Build history of the part. All positions in model axes, mm. A direction names the side the tool comes from. Round coordinates to 2 decimals unless told otherwise and drop trailing zeros. Loops run counter-clockwise (first coordinate to the right, second up) from the corner with the lowest first, then second, coordinate; pieces in that order, holes last. Notation, with made-up numbers: (57, 2.25) - (76, 2.25) arc R15 cw to (76, 20.25) - close; hole circle Ø6 at (-37, 17). An arc over 180 degrees is marked (long way). Put each result on its own line as item: value. Start each with the question number.
Autodesk Fusion 360 part; units mm, degrees
sketch "Esquisse1" plane through (0, 0, 0) normal (0, 1, 0) x (1, 0, 0)
  line L0 (0, 0) -> (150, 0)
  line L1 (150, 0) -> (150, -35)
  line L2 (150, -35) -> (0, -35)
  line L3 (0, -35) -> (0, 0)
  line L4 (75, -35) -> (75, -60) construction
  line L5 (0, 0) -> (150, 0)
  line L6 (150, 0) -> (150, 2.5)
  line L7 (150, 2.5) -> (0, 2.5)
  line L8 (0, 2.5) -> (0, 0)
  line L9 (150, -35) -> (152.5, -35)
  line L10 (152.5, -35) -> (152.5, 2.5)
  line L11 (152.5, 2.5) -> (150, 2.5)
  line L12 (150, 2.5) -> (150, -35)
  line L13 (0, -35) -> (-2.5, -35)
  line L14 (-2.5, -35) -> (-2.5, 2.5)
  line L15 (-2.5, 2.5) -> (0, 2.5)
  line L16 (0, 2.5) -> (0, -35)
  line L17 (-2.5, -35) -> (71.93, -59.0097)
  line L18 (78.07, -59.0097) -> (152.5, -35)
  arc A0 (71.93, -59.0097) -> (78.07, -59.0097) centre (75, -49.4926) ccw
  point P0 (75, -35)
  dimension "d6" = 150
  dimension "d7" = 35
  dimension "d8" = 25
  dimension "d13" = 150
  dimension "d14" = 2.5
  dimension "d15" = 2.5
  dimension "d16" = 37.5
  dimension "d17" = 2.5
  dimension "d18" = 37.5
  dimension "d19" = 10
extrude "Extrusion2" add sketch "Esquisse1" along normal blind 2.5 contours L0 L1 L2 L3 L5 L12 L16 | L2 L9 L13 L17 L18 A0
extrude "Extrusion3" add sketch "Esquisse1" along normal blind 70 contours L0 L5 L6 L7 L8 L12 L16 | L3 L8 L13 L14 L15 L16 | L1 L6 L9 L10 L11 L12
ref_plane "Plan de construction1" through (75, 70, 16.25) normal (0, 1, 0) x (0, 0, 1)
sketch "Esquisse2" plane through (75, 70, 16.25) normal (0, 1, 0) x (1, 0, 0)
  line L0 (-75, 16.25) -> (-75, -18.75)
  line L1 (-75, -18.75) -> (-77.5, -18.75)
  line L2 (-77.5, -18.75) -> (-3.07, -42.7597)
  arc A0 (-3.07, -42.7597) -> (3.07, -42.7597) centre (0, -33.2426) ccw
  line L3 (3.07, -42.7597) -> (77.5, -18.75)
  line L4 (77.5, -18.75) -> (75, -18.75)
  line L5 (75, -18.75) -> (75, 16.25)
  line L6 (75, 16.25) -> (-75, 16.25)
  line L7 (75, -18.75) -> (-75, -18.75)
  line L8 (-75, -18.75) -> (-75, 16.25)
  line L9 (-75, 16.25) -> (75, 16.25)
  line L10 (75, 16.25) -> (75, -18.75)
  line L11 (75, -1.25) -> (-75, -1.25) construction
  line L12 (75, -1.25) -> (25, -1.25) construction
  line L13 (-75, -1.25) -> (-25, -1.25) construction
  circle A1 centre (25, -1.25) radius 2.25
  circle A2 centre (-25, -1.25) radius 2.25
  point P0 (75, -1.25)
  point P1 (-75, -1.25)
  dimension "d27" = 50
  dimension "d28" = 50
  dimension "d30" = 4.5
  dimension "d31" = 4.5
extrude "Extrusion4" add sketch "Esquisse2" against normal blind 2.5 contours L0 L5 L6 L7 L8 L9 L10 | A1 | A2
extrude "Extrusion5" cut sketch "Esquisse2" against normal blind 2.5 contours A1 | A2
equation "bagWidth = 150 mm"
equation "bagThickness = 65 mm"
equation "dispenserBorderHeight = 35 mm"
equation "dispenserTriangleHeight = 25 mm"
equation "dispenserThickness = 2.5 mm"
equation "d6 = bagWidth"
equation "d7 = dispenserBorderHeight"
equation "d8 = dispenserTriangleHeight"
equation "dispenserTriangleRoundCorner = 10 mm"
equation "d13 = bagWidth"
equation "d14 = dispenserThickness"
equation "d15 = dispenserThickness"
equation "d16 = dispenserBorderHeight + dispenserThickness"
equation "d17 = dispenserThickness"
equation "d18 = dispenserBorderHeight + dispenserThickness"
equation "d19 = dispenserTriangleRoundCorner"
equation "d20 = dispenserThickness"
equation "d22 = ( 2 * dispenserThickness ) + bagThickness"
equation "d27 = bagWidth / 3"
equation "d28 = bagWidth / 3"
equation "screwHoleDiameter = 4.5 mm"
equation "d30 = screwHoleDiameter"
equation "d31 = screwHoleDiameter"
1) Slice it at C-C, the plane y = 24. Write the cut outline in (x, z), and give its area (4 significant figures).
2) Slice it at D-D, the plane x = 13. Write the cut outline in (y, z).
3) Slice it at A-A, the plane z = 6. Write the cut outline in (x, y).
4) Drop flat-ended pins along their axis: pin 1 Ø3 at (x, y) = (26, 32.5) entering from +Z; pin 2 Ø3 at (x, z) = (57.5, 45) entering from +Y. Give the stop position or say it passes through.
5) Drill centre lines: line 1 (X direction, y = 68.95, z = 17.5); line 2 (Z direction, x = 100, y = 68.1); line 3 (Y direction, x = 146, z = 32.5). Where is each one in solid material? Low to high. Write a range as [from, to].
6) Pull direction X, two halves, no side cores. Call faces 1 (the face through (76, 35, -2.5)), 2 (the face through (34.194, 1.232, 46.837)), 3 (the face through (114.764, 1.232, 47.173)), 4 (the face through (150, 35, 17)): pulls with the +X half, pulls with the -X half, needs draft (parallel to the pull), parting line crosses it, or undercut.
7) Slice it at B-B, the plane z = 17.5. Write the cut outline in (x, y), and give its area (3 significant figures).
8) Which spindle directions (+Z, -Z, +X, -X, +Y, -Y) get a long thin tool onto all of the face, cutting with end or side? Do faces 5 (the face through (75, 69, 35)), 6 (the face through (48.214, 68.768, 18.869)), 7 (the face through (0, 35, 18)). Say none if no direction does.
Taken from the geometry:
1. outline: (-2.5, -2.5) - (152.5, -2.5) - (152.5, 35) - (150, 35) - (150, 0) - (0, 0) - (0, 35) - (-2.5, 35) - close
1. area: 562.5 mm2
2. outline: (0, -2.5) - (70, -2.5) - (70, 35) - (67.5, 35) - (67.5, 0) - (2.5, 0) - (2.5, 40) - (0, 40) - close
3. outline: (-2.5, 0) - (152.5, 0) - (152.5, 70) - (-2.5, 70) - close; hole (0, 2.5) - (150, 2.5) - (150, 67.5) - (0, 67.5) - close
4. pin 1: stops at z = 0
4. pin 2: stops at y = 2.5
5. line 1: x = [-2.5, 47.75], [52.25, 97.75], [102.25, 152.5]
5. line 2: z = [-2.5, 15.25], [19.75, 35]
5. line 3: y = [0, 2.5], [67.5, 70]
6. face 1: needs draft
6. face 2: pulls with the -X half
6. face 3: pulls with the +X half
6. face 4: undercut
7. outline: (-2.5, 0) - (152.5, 0) - (152.5, 70) - (102.25, 70) - (102.25, 67.5) - (150, 67.5) - (150, 2.5) - (0, 2.5) - (0, 67.5) - (47.75, 67.5) - (47.75, 70) - (-2.5, 70) - close; (52.25, 67.5) - (97.75, 67.5) - (97.75, 70) - (52.25, 70) - close
7. area: 1,080 mm2
8. face 5: +Z, +X, -X, +Y
8. face 6: +Y
8. face 7: +Z
